Work out the finished part from the listing and answer in its coordinate system (mm). A direction names the side the tool comes from. Coordinates: 2 decimals unless noted, no trailing zeros. Order: outer loops, then holes, each group sorted by start corner. A loop starts at its lowest first (then second) coordinate and runs counter-clockwise, first axis right, second up. Notation, with made-up numbers: M 50.5,67 L 92.5,67 A7 cw 92.5,80 Z; hole C -37.5,15 d2. An arc over 180 degrees is marked long. Answer in a Markdown table with one row per item. Add a question column.
Item 1: Flat-ended cylindrical pins translate along their axes: pin 1 Ø0.7 at (y, z) = (1.5, 1.5) entering from +X; pin 2 Ø1 at (x, y) = (-14.5, -1.5) entering from +Z; pin 3 Ø1.1 at (x, z) = (-11.5, 0.5) entering from +Y. Find the tip coordinate at first contact, or state that the pin passes through.
Item 2: Consider line 1 (X direction, y = -4.5, z = 2); line 2 (Y direction, x = -6.75, z = 2.25); line 3 (Z direction, x = -19.75, y = -0.25). Determine where each line is inside the solid, lowest interval first. Write a range as from..to.
Item 3: The part is cut by section C-C (y = -2.5). Write down the section's boundary in (x, z).
Item 4: The part is cut by section B-B (z = 2). State how many separate pieces and enclosed holes the cut face has, then the cut area to 3 significant figures.
Item 5: The part is cut by section A-A (x = -9). Write down the section's boundary in (y, z).
Item 6: The mould has two halves that part along Y. Classify faces 1 (the face through (-20, -4.041, 2)), 2 (the face through (-13, 2.459, 1)), 3 (the face through (-17.68, 2, 1)): released by +Y, released by -Y, zero draft, split by the parting line, or undercut.
Item 7: Which of the six approach directions +Z, -Z, +X, -X, +Y, -Y give full straight-line access (tool end or side, diameter ignored) to faces 4 (the face through (-6.88, -5, 1)), 5 (the face through (-14.08, 2, 1)), 6 (the face through (-5.08, 2, 1)), 7 (the face through (-12, -2, 1))?
Item 8: The part is cut by section D-D (x = -11.25). Write down the section's boundary in (y, z).
from build123d import *

# Parameters (mm, degrees)
F1_DEPTH = 1
F0_W     = 1.8
F0_H     = 1.5
F2_DEPTH = 2.5


with BuildPart() as f1:
    # F0 (on Top) → F1 (new body)
    with BuildSketch(Plane.XY):
        Polygon((-19.480222, 0.959121), (-21.280222, 0.959121), (-21.280222, -0.040879), (-21.280222, -3.040879), (-21.280222, -4.040879), (-19.480222, -4.040879), (-17.680222, -4.040879), (-15.880222, -4.040879), (-14.080222, -4.040879), (-12.280222, -4.040879), (-10.480222, -4.040879), (-8.680222, -4.040879), (-6.880222, -4.040879), (-5.080222, -4.040879), (-3.280222, -4.040879), (-3.280222, -3.040879), (-3.280222, -0.040879), (-3.280222, 0.959121), (-5.080222, 0.959121), (-6.880222, 0.959121), (-8.680222, 0.959121), (-10.480222, 0.959121), (-12.280222, 0.959121), (-14.080222, 0.959121), (-15.880222, 0.959121), (-17.680222, 0.959121), align=None)
    extrude(amount=F1_DEPTH)

    # F0 (on Top) → F2 (join)
    with BuildSketch(Plane.XY):
        with Locations((-20.380222, 1.709121)):
            Rectangle(F0_W, F0_H)
        with Locations((-16.780222, 1.709121)):
            Rectangle(F0_W, F0_H)
        with Locations((-13.180222, 1.709121)):
            Rectangle(F0_W, F0_H)
        with Locations((-9.580222, 1.709121)):
            Rectangle(F0_W, F0_H)
        with Locations((-5.980222, 1.709121)):
            Rectangle(F0_W, F0_H)
        with Locations((-5.980222, -4.790879)):
            Rectangle(F0_W, F0_H)
        with Locations((-9.580222, -4.790879)):
            Rectangle(F0_W, F0_H)
        with Locations((-13.180222, -4.790879)):
            Rectangle(F0_W, F0_H)
        with Locations((-16.780222, -4.790879)):
            Rectangle(F0_W, F0_H)
        with Locations((-20.380222, -4.790879)):
            Rectangle(F0_W, F0_H)
    extrude(amount=F2_DEPTH)


solid = f1.part
Reply:
| question | item | result |
|---|---|---|
| 1 | pin 1 | stops at x = -5.08 |
| 1 | pin 2 | stops at z = 1 |
| 1 | pin 3 | stops at y = 0.96 |
| 2 | line 1 | x = -21.28..-19.48, -17.68..-15.88, -14.08..-12.28, -10.48..-8.68, -6.88..-5.08 |
| 2 | line 2 | y = -5.54..-4.04, 0.96..2.46 |
| 2 | line 3 | z = 0..1 |
| 3 | outline | M -21.28,0 L -3.28,0 L -3.28,1 L -21.28,1 Z |
| 4 | separate pieces | 10 |
| 4 | enclosed holes | 0 |
| 4 | area | 27.0 mm2 |
| 5 | outline | M -5.54,0 L 2.46,0 L 2.46,2.5 L 0.96,2.5 L 0.96,1 L -4.04,1 L -4.04,2.5 L -5.54,2.5 Z |
| 6 | face 1 | undercut |
| 6 | face 2 | released by +Y |
| 6 | face 3 | zero draft |
| 7 | face 4 | +Z, -Z, -Y |
| 7 | face 5 | +Z, -Z, +Y |
| 7 | face 6 | +Z, -Z, +X, +Y |
| 7 | face 7 | +Z, +X, -X |
| 8 | outline | M -4.04,0 L 0.96,0 L 0.96,1 L -4.04,1 Z |
